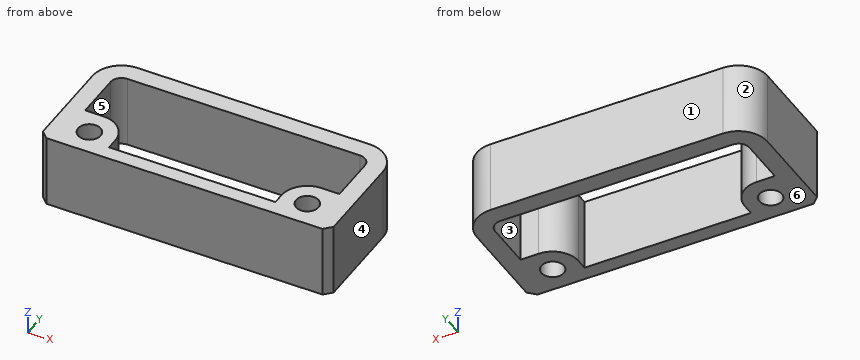
```python
from build123d import *

# Parameters (mm, degrees)
F0_R     = 1.55
F1_DEPTH = 10
F3_SIZE  = 1


with BuildPart() as f1:
    # F0 (on Top) → F1 (new body)
    with BuildSketch(Plane.XY):
        with BuildLine():
            Line((16, 17.55), (0, 17.55))
            Line((0, 17.55), (0, 15.05))
            Line((0, 15.05), (16, 15.05))
            ThreePointArc((16, 15.05), (17.0606601718, 14.6106601718), (17.5, 13.55))
            Line((17.5, 13.55), (17.5, 7.1))
            Line((17.5, 7.1), (15, 7.1))
            ThreePointArc((15, 7.1), (12.4897709268, 6.0602290732), (11.45, 3.55))
            Line((11.45, 3.55), (11.45, 2))
            Line((11.45, 2), (0, 2))
            Line((0, 2), (0, 0))
            Line((0, 0), (20, 0))
            Line((20, 0), (20, 13.55))
            ThreePointArc((20, 13.55), (18.8284271247, 16.3784271247), (16, 17.55))
        make_face()
        with Locations((15, 3.55)):
            Circle(F0_R, mode=Mode.SUBTRACT)
    extrude(amount=F1_DEPTH)

    # F2: F1 across face


with BuildPart() as f1_1:
    add(f1.part)
    add(f1.part.mirror(Plane(origin=(0, 16.3, 5), x_dir=(0, -1, 0), z_dir=(-1, 0, 0))))

    # F3
    f3_edges = [f1_1.edges().sort_by_distance(p)[0] for p in [
        (-20, 0, 5),
        (20, 0, 5),
    ]]
    chamfer(f3_edges, length=F3_SIZE)


solid = f1_1.part
```
Build history of the part. All positions in model axes, mm. Face numbers are marked on the shaded views. A direction names the side the tool comes from. Give positions to 0.01 mm unless a question says otherwise; leave off trailing zeros. Loops run counter-clockwise (first coordinate to the right, second up) from the corner with the lowest first, then second, coordinate; pieces in that order, holes last. Notation, with made-up numbers: (-36, -19.5) -> (-21, -19.5) arc R23 ccw to (-21, 5.5) -> close; hole circle Ø11 at (83.25, 26.5). An arc over 180 degrees is marked (long way). One line per question, with ' | ' between items.
Q1. Cut at C-C, the plane y = 6. Write the cut outline in (x, z).
Filled sheet:
outline: (-20, 0) -> (-12.43, 0) -> (-12.43, 10) -> (-20, 10) -> close; (12.43, 0) -> (20, 0) -> (20, 10) -> (12.43, 10) -> close
Q2. Cut at B-B, the plane x = -1. Write the cut outline in (y, z).
Filled sheet:
outline: (0, 0) -> (2, 0) -> (2, 10) -> (0, 10) -> close; (15.05, 0) -> (17.55, 0) -> (17.55, 10) -> (15.05, 10) -> close
Q3. Cut at A-A, the plane z = 9.5. Write the cut outline in (x, y), plus the area to 3 significant figures.
Filled sheet:
outline: (-20, 1) -> (-19, 0) -> (19, 0) -> (20, 1) -> (20, 13.55) arc R4 ccw to (16, 17.55) -> (-16, 17.55) arc R4 ccw to (-20, 13.55) -> close; hole (-17.5, 7.1) -> (-15, 7.1) arc R3.55 cw to (-11.45, 3.55) -> (-11.45, 2) -> (11.45, 2) -> (11.45, 3.55) arc R3.55 cw to (15, 7.1) -> (17.5, 7.1) -> (17.5, 13.55) arc R1.5 ccw to (16, 15.05) -> (-16, 15.05) arc R1.5 ccw to (-17.5, 13.55) -> close; hole circle Ø3.1 at (-15, 3.55); hole circle Ø3.1 at (15, 3.55) | area: 280 mm²
Q4. Drill centre lines: line 1 along Y through (x, z) = (-15, 5.5); line 2 along X through (y, z) = (11, 3.5); line 3 along Y through (x, z) = (-1.5, 7). Where is each one in solid material? Low to high. Write a range as [from, to].
Filled sheet:
line 1: y = [0, 2], [5.1, 7.1], [15.05, 17.55] | line 2: x = [-20, -17.5], [17.5, 20] | line 3: y = [0, 2], [15.05, 17.55]
Q5. Drop a flat-ended pin along its axis: pin 1 (2.5 mm diameter, centred on x = 15, y = 3.55, fed in from -Z). Give the stop position or say it passes through.
Filled sheet:
pin 1: passes through
Q6. Pull direction X, two halves, no side cores. Call the marked faces 1, 2, 3 and 4: pulls with the +X half, pulls with the -X half, needs draft (parallel to the pull), parting line crosses it, or undercut.
Filled sheet:
face 1: needs draft | face 2: pulls with the -X half | face 3: undercut | face 4: pulls with the +X half
Q7. Tool access for the marked faces 5 and 6: list every direction of +Z, -Z, +X, -X, +Y, -Y with a clear straight run to the whole face (end or side of a thin tool).
Filled sheet:
face 5: +Z, -Z | face 6: -Z, +X, -X, +Y, -Y
Q8. Cut at D-D, the plane y = 16.5. Write the cut outline in (x, z), plus the area to 3 significant figures.
Filled sheet:
outline: (-18.7, 0) -> (18.7, 0) -> (18.7, 10) -> (-18.7, 10) -> close | area: 374 mm²
